Geometry check sheet. Reference: the model listing, model coordinates, mm. A direction names the side the tool comes from. Round coordinates to 2 decimals unless told otherwise and drop trailing zeros. Order: outer loops, then holes, each group sorted by start corner. A loop starts at its lowest first (then second) coordinate and runs counter-clockwise, first axis right, second up. Notation, with made-up numbers: (69.5, 72) - (114.5, 72) arc R28 cw to (114.5, 100) - close; hole circle Ø9 at (83.25, -1.5). An arc over 180 degrees is marked (long way). Return JSON: item names as keys, results as strings. Group by question number.
Q1. Tool access check on faces 1 (the flat face through (108, 25, 0)), 2 (the flat face through (0, 25, 50)). Record the directions out of +Z, -Z, +X, -X, +Y, -Y that give a thin tool (end or side, any length) a straight path to the whole face; none if there is none.
Q2. Sectioned sample at B-B, the plane y = 25.4. Record the cut outline in (x, z) (3 decimals).
Q3. Sectioned sample at A-A, the plane z = 19.05. Record the cut outline in (x, y) (3 decimals).
Q4. Sectioned sample at D-D, the plane z = 60.5. Record the cut outline in (x, y), then the cut area to 3 significant figures.
Q5. Sectioned sample at C-C, the plane x = 50.8. Record the cut outline in (y, z) (3 decimals).
Q6. Material ranges on line 1 along Z through (x, y) = (107, 25.4) (3 decimals); line 2 along X through (y, z) = (3.5, 30.5); line 3 along Y through (x, z) = (50, 111), recorded low to high.
Q7. Draft check along Y on faces 3 (the flat face through (46, 50.8, 104)), 4 (the cylindrical face through (-6.261, 17.841, 13.254)), 5 (the flat face through (-6, 25, 0)), 6 (the cylindrical face through (55.2, 16.95, 108.04)). Enter one of: pulls with the +Y half, pulls with the -Y half, needs draft (parallel to the pull), parting line crosses it, or undercut.
Q8. Gauge pin test, flat ends, axial feed: pin 1 Ø8 at (x, y) = (62, 35.5) entering from -Z; pin 2 Ø17 at (x, y) = (50.8, 25.4) entering from +Z. Record the tip position at first contact, or that the pin passes through.
```python
from build123d import *

# Parameters (mm, degrees)
F1_DEPTH = 50.8
F2_R     = 9.525
F3_DEPTH = 127
F4_R     = 9.525
F5_DEPTH = 12.7


with BuildPart() as f1:
    # F0 (on Front) → F1 (new body)
    with BuildSketch(Plane.XZ):
        Polygon((-12.7, 0), (0, 0), (0, 101.6), (101.6, 101.6), (101.6, 0), (114.3, 0), (114.3, 114.3), (-12.7, 114.3), align=None)
    extrude(amount=-F1_DEPTH)

    # F2 (on face) → F3 (cut)
    with BuildSketch(Plane.YZ.offset(114.3)):
        with Locations((25.4, 19.05)):
            Circle(F2_R)
    extrude(amount=-F3_DEPTH, mode=Mode.SUBTRACT)

    # F4 (on face) → F5 (cut, through all)
    with BuildSketch(Plane.XY.offset(114.3)):
        with Locations((50.8, 25.4)):
            Circle(F4_R)
    extrude(amount=-F5_DEPTH, mode=Mode.SUBTRACT)


solid = f1.part
```
Reply:
{
 "1": {"face 1": "-Z, +X, -X, +Y, -Y", "face 2": "-Z, +Y, -Y"},
 "2": {"outline": "(-12.7, 0) - (0, 0) - (0, 9.525) - (-12.7, 9.525) - close; (-12.7, 28.575) - (0, 28.575) - (0, 101.6) - (41.275, 101.6) - (41.275, 114.3) - (-12.7, 114.3) - close; (60.325, 101.6) - (101.6, 101.6) - (101.6, 28.575) - (114.3, 28.575) - (114.3, 114.3) - (60.325, 114.3) - close; (101.6, 0) - (114.3, 0) - (114.3, 9.525) - (101.6, 9.525) - close"},
 "3": {"outline": "(-12.7, 0) - (0, 0) - (0, 15.875) - (-12.7, 15.875) - close; (-12.7, 34.925) - (0, 34.925) - (0, 50.8) - (-12.7, 50.8) - close; (101.6, 0) - (114.3, 0) - (114.3, 15.875) - (101.6, 15.875) - close; (101.6, 34.925) - (114.3, 34.925) - (114.3, 50.8) - (101.6, 50.8) - close"},
 "4": {"outline": "(-12.7, 0) - (0, 0) - (0, 50.8) - (-12.7, 50.8) - close; (101.6, 0) - (114.3, 0) - (114.3, 50.8) - (101.6, 50.8) - close", "area": "1,290 mm^2"},
 "5": {"outline": "(0, 101.6) - (15.875, 101.6) - (15.875, 114.3) - (0, 114.3) - close; (34.925, 101.6) - (50.8, 101.6) - (50.8, 114.3) - (34.925, 114.3) - close"},
 "6": {"line 1": "0 to 9.525, 28.575 to 114.3", "line 2": "-12.7 to 0, 101.6 to 114.3", "line 3": "0 to 15.91, 34.89 to 50.8"},
 "7": {"face 3": "pulls with the +Y half", "face 4": "undercut", "face 5": "needs draft", "face 6": "undercut"},
 "8": {"pin 1": "z = 101.6", "pin 2": "through"}
}
